Can you work these out from the model? Positions are in its coordinate system, mm. A direction names the side the tool comes from. Give positions to 0.01 mm unless a question says otherwise; leave off trailing zeros. Loops run counter-clockwise (first coordinate to the right, second up) from the corner with the lowest first, then second, coordinate; pieces in that order, holes last. Notation, with made-up numbers: M 16,-33.75 L 65,-33.75 A36 ccw 65,4.25 Z; hole C -20,-19.75 d7. An arc over 180 degrees is marked long. Put each result on its own line as item: value. Start each with the question number.
1) Please list where these lines run through material, in increasing order: line 1 along X through (y, z) = (2, -1.35); line 2 along Y through (x, z) = (1.1, -1.3). Write a range as from..to.
2) For P1, Ø1.7, axis at x = 2, y = 2, coming from the +Z side; P2, Ø1, axis at x = 1, z = -2.5, coming from the -Y side, each with a flat end and sliding along its axis, tell me the tip position at first contact or that it passes through.
3) Imagine slicing it at D-D (y = 1.5). Write out the boundary of the cut face in (x, z).
4) If we mould it in two halves opening along X, with no side actions, what happens to faces 3 (the cylindrical face through (3.43, 0.6, -2.54)), 4 (the cylindrical face through (0.57, 0.6, -2.46)), 5 (the flat face through (2, 4, -2))? For each: +X half, -X half, draft (parallel to the pull), parting line (faces both ways), or undercut.
5) For faces 1 (the flat face through (3.5, 5, -2)), 2 (the flat face through (0, 4, -3)), which set-ups out of +Z, -Z, +X, -X, +Y, -Y let a thin tool reach every point of the face, with its end or its side?
6) Imagine slicing it at C-C (x = 1.2). Write out the boundary of the cut face in (y, z), then the cut area to 3 significant figures.
Autodesk Inventor part; units mm, degrees
ref_plane "YZ Plane" through (0, 0, 0) normal (1, 0, 0) x (0, 1, 0)
ref_plane "XZ Plane" through (0, 0, 0) normal (0, 1, 0) x (-1, 0, 0)
ref_plane "XY Plane" through (0, 0, 0) normal (0, 0, 1) x (1, 0, 0)
sketch "スケッチ1" plane through (0, 0, 0) normal (0, 1, 0) x (-1, 0, 0)
  line L0 (0, 0) -> (-4, 0)
  line L1 (-4, 0) -> (-4, -5)
  line L2 (-4, -5) -> (0, -5)
  line L3 (0, -5) -> (0, 0)
  dimension "d0" = 4
  dimension "d1" = 5
extrude "押し出し1" add sketch "スケッチ1" along normal blind 6.5
sketch "スケッチ2" plane through (0, 0, 0) normal (0, 0, 1) x (1, 0, 0)
  line L0 (0, 0) -> (4, 0)
  line L1 (0, 0) -> (0, 6.5)
  point P0 (2, 2)
  dimension "d11" = 2
  dimension "d12" = 2
hole "穴1" at (2, 2, 0) direction (0, 0, -1) diameter 2.1 end through all
sketch "スケッチ3" plane through (0, 0, 0) normal (0, 0, 1) x (1, 0, 0)
  line L0 (0.5, 6.5) -> (3.5, 6.5)
  line L1 (3.5, 6.5) -> (3.5, 4)
  line L2 (3.5, 4) -> (0.5, 4)
  line L3 (0.5, 4) -> (0.5, 6.5)
  line L4 (0.5, 6.5) -> (3.5, 4) construction
  line L5 (3.5, 6.5) -> (0.5, 4) construction
  line L6 (0, 0) -> (0, 6.5)
  line L7 (0, 6.5) -> (4, 6.5)
  point P0 (2, 5.25)
  dimension "d13" = 3
  dimension "d14" = 2.5
  dimension "d15" = 2
  dimension "d16" = 0
extrude "押し出し2" cut sketch "スケッチ3" against normal through all
fillet "フィレット1" radius 2 2 edges at (4, 0, -2.5) (0, 0, -2.5)
fillet "フィレット2" radius 0.5 4 edges at (0.5, 5.25, 0) (3.5, 5.25, 0) (0.5, 5.25, -5) (3.5, 5.25, -5)
properties part number "gomu_guide"
Recorded:
1. line 1: 0..0.95, 3.05..4
1. line 2: 0.21..1.46, 2.54..4
2. P1: through
2. P2: y = 0.06
3. outline: M 0.06,-5 L 1.08,-5 L 1.08,0 L 0.06,0 Z; M 2.92,-5 L 3.94,-5 L 3.94,0 L 2.92,0 Z
4. face 3: +X half
4. face 4: -X half
4. face 5: undercut
5. face 1: +Z, -Z, +Y
5. face 2: +Z, -Z, -X, +Y, -Y
6. outline: M 0.17,-5 L 1.32,-5 L 1.32,0 L 0.17,0 Z; M 2.68,-5 L 4,-5 L 4,0 L 2.68,0 Z
6. area: 12.4 mm²
